For this review, use the dimensioned drawing (mm, ordinates from the lowest corner) and the shaded views. Round coordinates to 2 decimals unless told otherwise and drop trailing zeros. Loops run counter-clockwise (first coordinate to the right, second up) from the corner with the lowest first, then second, coordinate; pieces in that order, holes last. Notation, with made-up numbers: (-6.5, -6.75) - (52.5, -6.75) arc R20 cw to (52.5, 6.25) - close; hole circle Ø7 at (76, 56.5). An arc over 180 degrees is marked (long way). Answer as CSV lines item,"result". Start each with the question number.
(1) Wall thickness on L1, parallel to Y at x = 15, z = 0.85; L2, parallel to Y at x = 11.5, z = 2.2: over which ranges is each line inside the solid? List them lowest first.
(2) Consider section A-A (x = 15). Give the boundary of the cut face in (y, z), and give its area (3 significant figures).
(3) Consider section B-B (y = 85). Give the boundary of the cut face in (x, z).
(4) Consider section C-C (z = 2.45). Give the boundary of the cut face in (x, y), and give its area (3 significant figures).
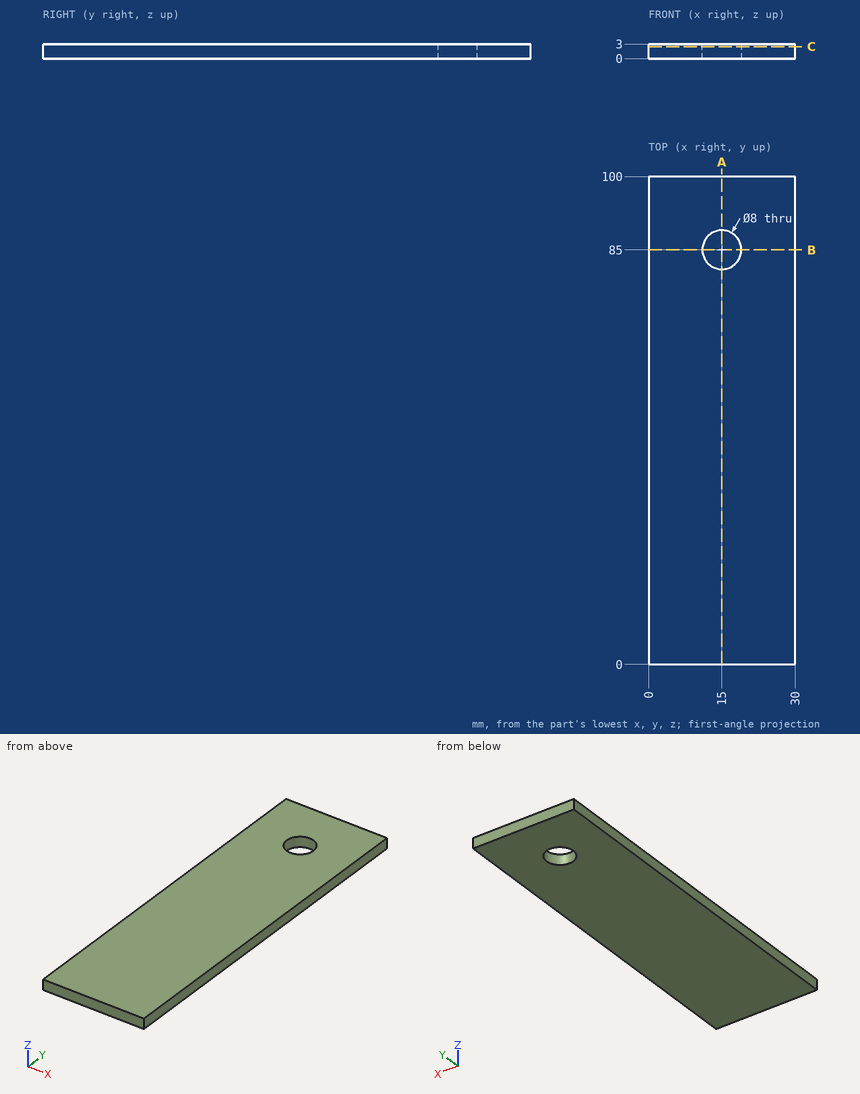
Determined:
1,L1,"y = 0 to 81, 89 to 100"
1,L2,"y = 0 to 83.06, 86.94 to 100"
2,outline,"(0, 0) - (81, 0) - (81, 3) - (0, 3) - close; (89, 0) - (100, 0) - (100, 3) - (89, 3) - close"
2,area,"276 mm^2"
3,outline,"(0, 0) - (11, 0) - (11, 3) - (0, 3) - close; (19, 0) - (30, 0) - (30, 3) - (19, 3) - close"
4,outline,"(0, 0) - (30, 0) - (30, 100) - (0, 100) - close; hole circle Ø8 at (15, 85)"
4,area,"2,950 mm^2"
